Geometry check sheet. Reference: drawing and pictorial views, mm from the part's lowest x, y, z. Coordinates: 2 decimals unless noted, no trailing zeros. Loops run counter-clockwise (first coordinate to the right, second up) from the corner with the lowest first, then second, coordinate; pieces in that order, holes last.
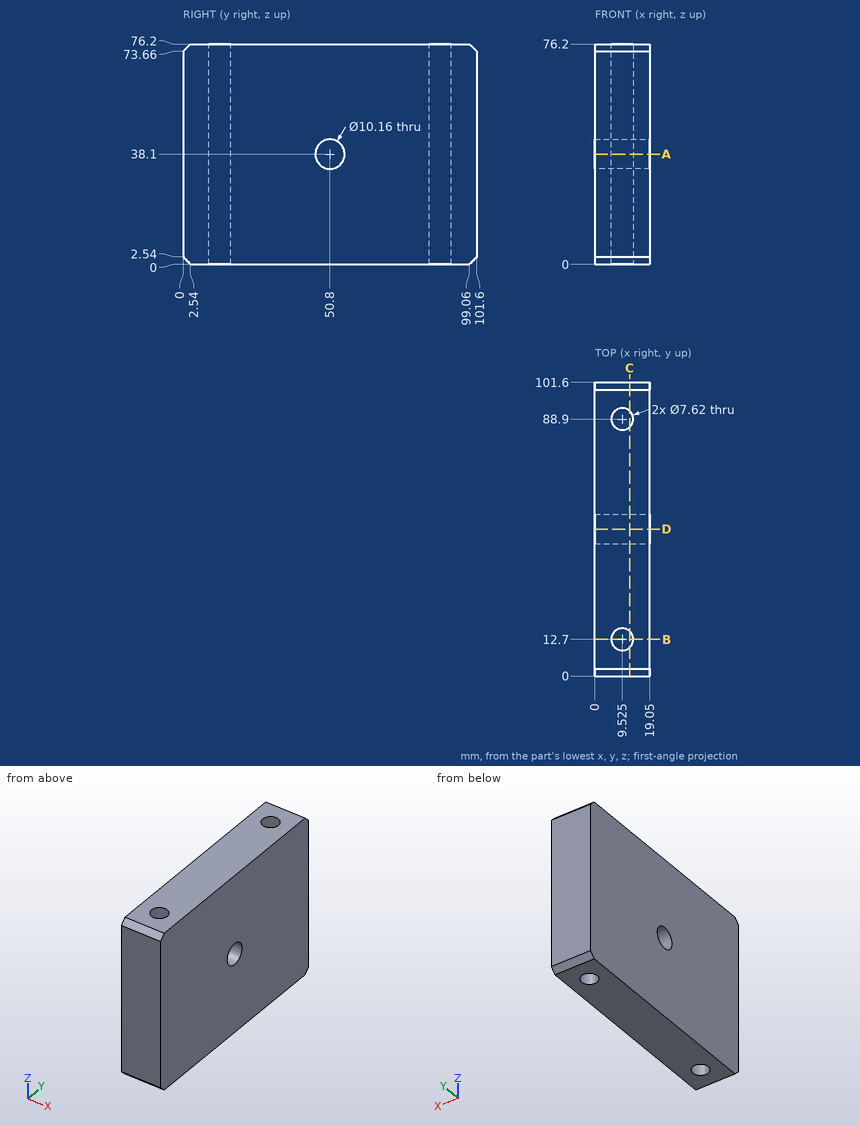
1) Section check B-B on y = 12.7. Record the cut outline in (x, z) (3 decimals), and give its area (3 significant figures).
Data:
outline: (0, 0) - (5.715, 0) - (5.715, 76.2) - (0, 76.2) - close; (13.335, 0) - (19.05, 0) - (19.05, 76.2) - (13.335, 76.2) - close
area: 871 mm2
2) Section check A-A on z = 38.1. Record the cut outline in (x, y) (3 decimals), and give its area (3 significant figures).
Data:
outline: (0, 0) - (19.05, 0) - (19.05, 45.72) - (0, 45.72) - close; (0, 55.88) - (19.05, 55.88) - (19.05, 101.6) - (0, 101.6) - close; hole circle Ø7.62 at (9.525, 12.7); hole circle Ø7.62 at (9.525, 88.9)
area: 1,650 mm2
3) Section check C-C on x = 12. Record the cut outline in (y, z), and give its area (3 significant figures).
Data:
outline: (0, 2.54) - (2.54, 0) - (9.8, 0) - (9.8, 76.2) - (2.54, 76.2) - (0, 73.66) - close; (15.6, 0) - (86, 0) - (86, 76.2) - (15.6, 76.2) - close; (91.8, 0) - (99.06, 0) - (101.6, 2.54) - (101.6, 73.66) - (99.06, 76.2) - (91.8, 76.2) - close; hole circle Ø10.16 at (50.8, 38.1)
area: 6,770 mm2
4) Depth check by flat-ended pin: pin 1 (6 mm diameter, centred on y = 50.8, z = 38.1, fed in from -X). Enter the tip coordinate at first touch or a pass-through.
Data:
pin 1: passes through
5) Section check D-D on y = 50.8. Record the cut outline in (x, z), and give its area (3 significant figures).
Data:
outline: (0, 0) - (19.05, 0) - (19.05, 33.02) - (0, 33.02) - close; (0, 43.18) - (19.05, 43.18) - (19.05, 76.2) - (0, 76.2) - close
area: 1,260 mm2
6) Material ranges on probe 1 along Y at (x, z) = (10, 52.5); probe 2 along Y at (x, z) = (7.5, 14.5); probe 3 along Z at (x, y) = (11, 50.5), recorded low to high.
Data:
probe 1: y = 0 to 8.92, 16.48 to 85.12, 92.68 to 101.6
probe 2: y = 0 to 9.47, 15.93 to 85.67, 92.13 to 101.6
probe 3: z = 0 to 33.03, 43.17 to 76.2
